Build history of the part. All positions in model axes, mm. Give positions to 0.01 mm unless a question says otherwise; leave off trailing zeros. Write each loop counter-clockwise with the first axis right and the second up, starting at its lowest first coordinate (ties: lowest second). Pieces come first, ordered by that corner, then holes. Notation, with made-up numbers: (30, 40.25) - (36, 40.25) arc R34 ccw to (36, 74.25) - close; hole circle Ø10 at (82, -16.75). An arc over 180 degrees is marked (long way). Use one line per item in the form item = value. Start each with the question number.
from build123d import *

# Parameters (mm, degrees)
SALIENTE_EXTRUIR1_DEPTH      = 3
SALIENTE_EXTRUIR1_DEPTH_BACK = 3
CROQUIS1_W                   = 20
CROQUIS1_H                   = 20
CROQUIS2_R                   = 0.9375
CORTAR_EXTRUIR4_DEPTH        = 0.1
MATRIZL1_COUNT               = 8
MATRIZL1_PITCH               = 2.5
MATRIZL1_COUNT_DIR2          = 8
MATRIZL1_PITCH_DIR2          = 2.5
CROQUIS4_R                   = 0.25
SALIENTE_EXTRUIR2_DEPTH      = 6
MATRIZL2_COUNT               = 8
MATRIZL2_PITCH               = 2.54
MATRIZL2_COUNT_DIR2          = 2
MATRIZL2_PITCH_DIR2          = 17.4625


with BuildPart() as part:
    # Croquis1 → Saliente-Extruir1 (new, two sides: drawn at the far end of the back side and taken through both)
    with BuildSketch(Plane(origin=(0, 0, 0), x_dir=(1, 0, 0), z_dir=(0, 1, 0)).offset(-SALIENTE_EXTRUIR1_DEPTH_BACK)):
        Rectangle(CROQUIS1_W, CROQUIS1_H)
    extrude(amount=SALIENTE_EXTRUIR1_DEPTH + SALIENTE_EXTRUIR1_DEPTH_BACK)

    # Croquis2 → Cortar-Extruir4 (cut)
    with BuildSketch(Plane(origin=(0, 3, 0), x_dir=(1, 0, 0), z_dir=(0, 1, 0))):
        with Locations(Location((-8.75, 8.75, 0), (0, 0, 270))):
            Circle(CROQUIS2_R)
    cortar_extruir4 = extrude(amount=-CORTAR_EXTRUIR4_DEPTH, mode=Mode.SUBTRACT)

    # MatrizL1: Cortar-Extruir4 8 × 8
    with Locations(*[(i * MATRIZL1_PITCH, 0, j * MATRIZL1_PITCH_DIR2) for i in range(MATRIZL1_COUNT) for j in range(MATRIZL1_COUNT_DIR2) if (i, j) != (0, 0)]):
        add(cortar_extruir4, mode=Mode.SUBTRACT)

    # Croquis4 → Saliente-Extruir2 (add)
    with BuildSketch(Plane(origin=(0, -3, 0), x_dir=(-1, 0, 0), z_dir=(0, -1, 0))):
        with Locations(Location((8.73125, -8.73125, 0), (0, 0, 270))):
            Circle(CROQUIS4_R)
    saliente_extruir2 = extrude(amount=SALIENTE_EXTRUIR2_DEPTH)

    # MatrizL2: Saliente-Extruir2 8 × 2
    with Locations(*[(i * MATRIZL2_PITCH, 0, -j * MATRIZL2_PITCH_DIR2) for i in range(MATRIZL2_COUNT) for j in range(MATRIZL2_COUNT_DIR2) if (i, j) != (0, 0)]):
        add(saliente_extruir2)


solid = part.part
(1) Cut at B-B, the plane z = -7.5. Give the cut face in (x, y), then the cut area to 3 significant figures.
(2) Two-plate mould, pull along X, no slides. Class faces 1 (the flat face through (-10, 0, 0)), 2 (the flat face through (-4, 2.9, 1)): +X half, -X half, draft (parallel to the pull), parting line (faces both ways), or undercut.
(3) Cut at A-A, the plane y = -6.5. State how many separate pieces and enclosed holes the cut face has, then the cut area to 3 significant figures.
(4) Wall check: line 1 (Y direction, x = -0.5, z = -3); line 2 (Y direction, x = 1.5, z = -3). Give the ranges that are in metal, low to high. Write a range as from..to.
(5) Pin check, flat tips, straight feed: pin 1 Ø1.5 at (x, z) = (1.5, -2) entering from -Y; pin 2 Ø1.5 at (x, z) = (-1.25, 3.75) entering from +Y; pin 3 Ø4 at (x, y) = (0.5, -7.5) entering from -Z. Stop position of each tip, or through.
Solution:
q1.outline = (-10, -3) - (10, -3) - (10, 3) - (-10, 3) - close
q1.area = 120 mm2
q2.face_1 = -X half
q2.face_2 = undercut
q3.separate_pieces = 16
q3.enclosed_holes = 0
q3.area = 3.14 mm2
q4.line_1 = -3..3
q4.line_2 = -3..2.9
q5.pin_1 = -3
q5.pin_2 = 2.9
q5.pin_3 = -8.98
